from build123d import *

# Parameters (mm, degrees)
BOSS_EXTRUDE1_DEPTH = 3.2004
SKETCH2_R           = 1.7272
SKETCH2_R_2         = 3.429
CUT_EXTRUDE1_DEPTH  = 3.2004
BOSS_EXTRUDE2_START = -3.2004
BOSS_EXTRUDE2_DEPTH = 3.2004
SKETCH4_R           = 6.35
CUT_EXTRUDE2_DEPTH  = 3.2004
FILLET1_R           = 12.7


with BuildPart() as part:
    # Sketch1 → Boss-Extrude1 (new body)
    with BuildSketch(Plane.XY):
        with BuildLine():
            ThreePointArc((-8.097097761, 15.832735205), (68.150612211, 34.198640293), (144.398322183, 15.832735205))
            ThreePointArc((144.398322183, 15.832735205), (152.133959628, -8.097097761), (128.204126662, -15.832735205))
            ThreePointArc((128.204126662, -15.832735205), (68.150612211, -1.367551307), (8.097097761, -15.832735205))
            ThreePointArc((8.097097761, -15.832735205), (-15.832735205, -8.097097761), (-8.097097761, 15.832735205))
        make_face()
    extrude(amount=BOSS_EXTRUDE1_DEPTH)

    # Sketch2 → Cut-Extrude1 (cut)
    with BuildSketch(Plane.XY.offset(3.2004)):
        with Locations((41.033365074, 11.300266799)):
            Circle(SKETCH2_R)
        with Locations((-9.725802761, 2.712083558)):
            Circle(SKETCH2_R)
        with Locations((-6.174081457, -6.6359257)):
            Circle(SKETCH2_R)
        with Locations((37.48164377, 20.648276058)):
            Circle(SKETCH2_R)
        with Locations((6.261836343, 3.437760818)):
            Circle(SKETCH2_R_2)
    extrude(amount=-CUT_EXTRUDE1_DEPTH, mode=Mode.SUBTRACT)

    # Sketch3 → Boss-Extrude2 (add)
    with BuildSketch(Plane.XY.offset(3.2004).offset(BOSS_EXTRUDE2_START)):
        with BuildLine():
            ThreePointArc((118.558560015, 1.198480685), (137.499705108, 17.742664408), (154.04388883, -1.198480685))
            ThreePointArc((154.04388883, -1.198480685), (151.248704167, -22.371604894), (145.781416871, -43.0167742))
            ThreePointArc((145.781416871, -43.0167742), (123.276823543, -54.242649292), (112.05094845, -31.738055964))
            ThreePointArc((112.05094845, -31.738055964), (116.357042584, -15.477699112), (118.558560015, 1.198480685))
        make_face()
    extrude(amount=BOSS_EXTRUDE2_DEPTH)

    # Sketch4 → Cut-Extrude2 (cut)
    with BuildSketch(Plane.XY.offset(3.2004)):
        with Locations((130.361522506, -37.860704571)):
            Circle(SKETCH4_R)
    extrude(amount=-CUT_EXTRUDE2_DEPTH, mode=Mode.SUBTRACT)

    # Fillet1
    fillet1_edges = [part.edges().sort_by_distance(p)[0] for p in [
        (117.190242121, -10.823434725, 1.6002),
    ]]
    fillet(fillet1_edges, radius=FILLET1_R)


solid = part.part
Could you check a few things on this model? Use its own coordinates, in mm. A direction names the side the tool comes from. Coordinates: 2 decimals unless noted, no trailing zeros. Write each loop counter-clockwise with the first axis right and the second up, starting at its lowest first coordinate (ties: lowest second). Pieces come first, ordered by that corner, then holes. Notation, with made-up numbers: M 22.5,53.5 L 46.5,53.5 A16 cw 46.5,67.5 Z; hole C -33.5,65 d7. An arc over 180 degrees is marked long. One line per question, with ' | ' between items.
1) I need wall thicknesses on probe 1 along Y at (x, z) = (130, 1.1); probe 2 along X at (y, z) = (-11.5, 2.7); probe 3 along X at (y, z) = (-13.5, 1.55). Which ranges of each line are inside material? Lowest first, please. Write a range as [from, to].
Checks:
probe 1: [-55.13, -44.2], [-31.52, 22.36] | probe 2: [-13.56, 17.45], [112.67, 153.03] | probe 3: [-11.58, 12.9], [113.91, 152.76]
2) Imagine slicing it at B-B, the plane z = 2. Give the number of separate pieces and of enclosed holes in the cut face, and give its area (3 significant figures).
Checks:
separate pieces: 1 | enclosed holes: 6 | area: 7,180 mm²
3) Imagine slicing it at A-A, the plane x = 127. Write out the boundary of the cut face in (y, z), and give its area (3 significant figures).
Checks:
outline: M -55.06,0 L -43.25,0 L -43.25,3.2 L -55.06,3.2 Z; M -32.47,0 L 23.52,0 L 23.52,3.2 L -32.47,3.2 Z | area: 217 mm²
4) For pin 1 Ø1.5 at (y, z) = (-38, 1) entering from +X; pin 2 Ø11.5 at (x, y) = (130.36, -37.86) entering from +Z, each with a flat end and sliding along its axis, tell me the tip position at first contact or that it passes through.
Checks:
pin 1: x = 147.59 | pin 2: through
5) If we mould it in two halves opening along X, with no side actions, what happens to faces 3 (the face through (123.649, -54.363, 1.578)), 4 (the face through (42.63, 10.64, 1.62)), 5 (the face through (69, 0, 3.2))? For each: released by +X, released by -X, zero draft, split by the parting line, or undercut.
Checks:
face 3: split by the parting line | face 4: undercut | face 5: zero draft
6) Imagine slicing it at C-C, the plane x = 23. Write out the boundary of the cut face in (y, z).
Checks:
outline: M -9.34,0 L 28,0 L 28,3.2 L -9.34,3.2 Z
7) For faces 1 (the face through (-7.45, -5.47, 1.62)), 2 (the face through (113.512, -27.084, 1.578)), which set-ups out of +Z, -Z, +X, -X, +Y, -Y let a thin tool reach every point of the face, with its end or its side?
Checks:
face 1: +Z, -Z | face 2: +Z, -Z, -X
8) Imagine slicing it at D-D, the plane x = 88. Write out the boundary of the cut face in (y, z), and give its area (3 significant figures).
Checks:
outline: M -2.87,0 L 33.02,0 L 33.02,3.2 L -2.87,3.2 Z | area: 115 mm²
